Verification items for this drawing (mm, ordinates from the low corner). A direction names the side the tool comes from. Coordinates: 2 decimals unless noted, no trailing zeros. Write each loop counter-clockwise with the first axis right and the second up, starting at its lowest first coordinate (ties: lowest second). Pieces come first, ordered by that corner, then holes. Notation, with made-up numbers: (25.25, 15) -> (54.25, 15) arc R34 ccw to (54.25, 49) -> close; hole circle Ø9 at (80, 77). An arc over 180 degrees is marked (long way). Use CSV: the item, a comma, the result in double quotes.
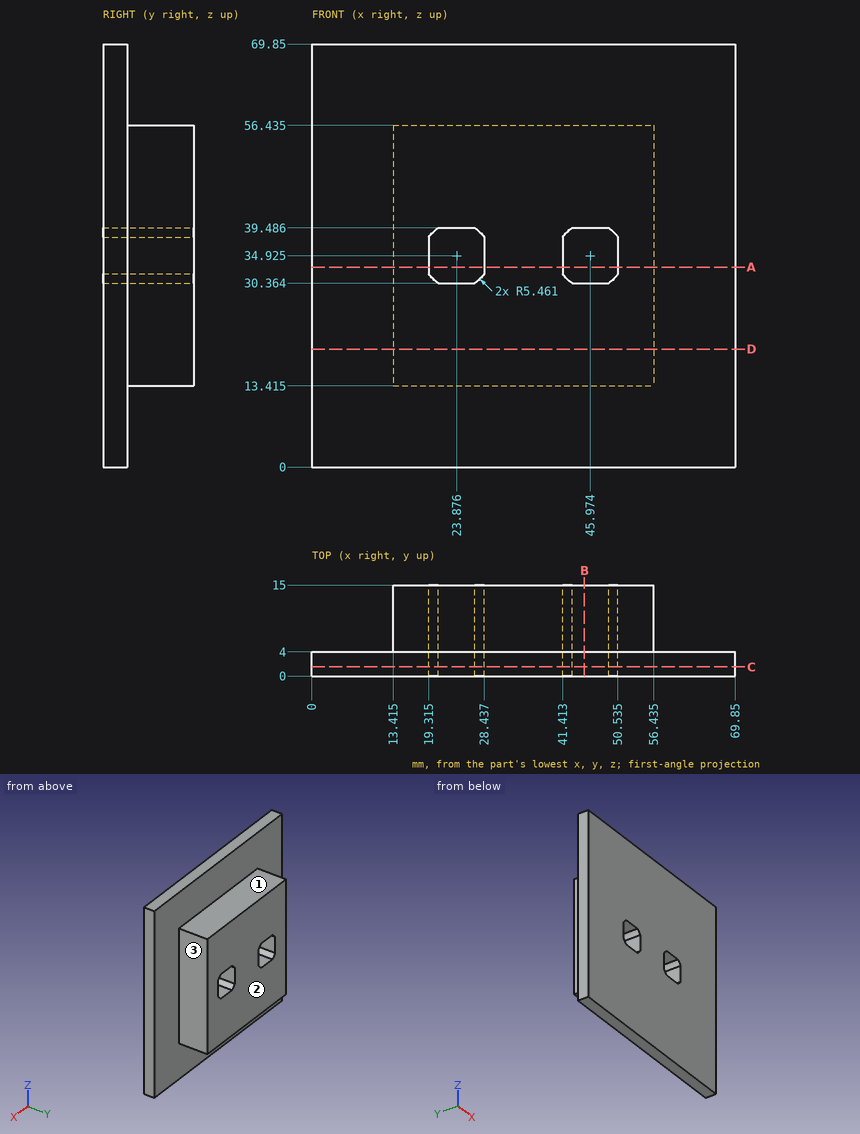
1) Cross-section at A-A (z = 33). Record the boundary of the cut face in (x, y) (3 decimals).
Return value:
outline,"(0, 0) -> (19.315, 0) -> (19.315, 15) -> (13.415, 15) -> (13.415, 4) -> (0, 4) -> close; (28.437, 0) -> (41.413, 0) -> (41.413, 15) -> (28.437, 15) -> close; (50.535, 0) -> (69.85, 0) -> (69.85, 4) -> (56.435, 4) -> (56.435, 15) -> (50.535, 15) -> close"
2) Cross-section at B-B (x = 45). Record the boundary of the cut face in (y, z) (3 decimals).
Return value:
outline,"(0, 0) -> (4, 0) -> (4, 13.415) -> (15, 13.415) -> (15, 30.364) -> (0, 30.364) -> close; (0, 39.486) -> (15, 39.486) -> (15, 56.435) -> (4, 56.435) -> (4, 69.85) -> (0, 69.85) -> close"
3) Cross-section at D-D (z = 19.5). Record the boundary of the cut face in (x, y) (3 decimals).
Return value:
outline,"(0, 0) -> (69.85, 0) -> (69.85, 4) -> (56.435, 4) -> (56.435, 15) -> (13.415, 15) -> (13.415, 4) -> (0, 4) -> close"
4) Cross-section at C-C (y = 1.5). Record the boundary of the cut face in (x, z) (3 decimals), plus the area to 3 significant figures.
Return value:
outline,"(0, 0) -> (69.85, 0) -> (69.85, 69.85) -> (0, 69.85) -> close; hole (19.315, 31.922) arc R5.461 ccw to (20.873, 30.364) -> (26.879, 30.364) arc R5.461 ccw to (28.437, 31.922) -> (28.437, 37.928) arc R5.461 ccw to (26.879, 39.486) -> (20.873, 39.486) arc R5.461 ccw to (19.315, 37.928) -> close; hole (41.413, 31.922) arc R5.461 ccw to (42.971, 30.364) -> (48.977, 30.364) arc R5.461 ccw to (50.535, 31.922) -> (50.535, 37.928) arc R5.461 ccw to (48.977, 39.486) -> (42.971, 39.486) arc R5.461 ccw to (41.413, 37.928) -> close"
area,"4,720 mm2"
5) Set-up check for the marked faces 1, 2 and 3: record each of +Z, -Z, +X, -X, +Y, -Y from which the full face is reachable in a straight line by a thin tool's end or side.
Return value:
face 1,"+Z, +X, -X, +Y"
face 2,"+Z, -Z, +X, -X, +Y"
face 3,"+Z, -Z, +X, +Y"
6) Scan lines: L1, parallel to X at y = 7.5, z = 34 (3 decimals); L2, parallel to Z at x = 26, y = 9 (3 decimals); L3, parallel to Y at x = 56.5, z = 30. Record each from-to range of solid material in increasing order.
Return value:
L1,"13.415 to 19.315, 28.437 to 41.413, 50.535 to 56.435"
L2,"13.415 to 30.364, 39.486 to 56.435"
L3,"0 to 4"
7) Gauge pin test, flat ends, axial feed: pin 1 (8 mm diameter, centred on y = 13, z = 22.5, fed in from -X) (3 decimals); pin 2 (5 mm diameter, centred on y = 8.5, z = 34.5, fed in from +X) (3 decimals); pin 3 (1.8 mm diameter, centred on x = 46, y = 10, fed in from +Z) (3 decimals); pin 4 (8 mm diameter, centred on x = 62.5, y = 9.5, fed in from +Z). Record the tip position at first contact, or that the pin passes through.
Return value:
pin 1,"x = 13.415"
pin 2,"x = 56.435"
pin 3,"z = 56.435"
pin 4,"through"
